from build123d import *

# Parameters (mm, degrees)
SKETCH1_R               = 32.5
BOSS_EXTRUDE1_DEPTH     = 3
CUT_EXTRUDE1_DEPTH      = 10
CUT_EXTRUDE1_DEPTH_BACK = 47.059743812
SKETCH2_W               = 5
SKETCH2_H               = 5


with BuildPart() as part:
    # Sketch1 → Boss-Extrude1 (new body)
    with BuildSketch(Plane(origin=(0, 0, 0), x_dir=(1, 0, 0), z_dir=(0, 1, 0))):
        with Locations(Location((0, 0, 0), (0, 0, 270))):
            Circle(SKETCH1_R)
    extrude(amount=BOSS_EXTRUDE1_DEPTH)

    # Sketch2 → Cut-Extrude1 (cut, two sides: drawn at the far end of the back side and taken through both)
    with BuildSketch(Plane(origin=(0, 0, 0), x_dir=(1, 0, 0), z_dir=(0, 1, 0)).offset(-CUT_EXTRUDE1_DEPTH_BACK)):
        with Locations((0, -27.5)):
            Rectangle(SKETCH2_W, SKETCH2_H)
        with Locations((27.5, 0)):
            Rectangle(SKETCH2_W, SKETCH2_H)
        with Locations((-27.5, 0)):
            Rectangle(SKETCH2_W, SKETCH2_H)
        with Locations((0, 27.5)):
            Rectangle(SKETCH2_W, SKETCH2_H)
    extrude(amount=CUT_EXTRUDE1_DEPTH + CUT_EXTRUDE1_DEPTH_BACK, mode=Mode.SUBTRACT)


solid = part.part
Geometry: final body of the model. Coordinates: model frame, mm. A direction names the side the tool comes from. Give positions to 0.01 mm unless a question says otherwise; leave off trailing zeros. Loops run counter-clockwise (first coordinate to the right, second up) from the corner with the lowest first, then second, coordinate; pieces in that order, holes last. Notation, with made-up numbers: M 42,13 L 88,13 A35 ccw 88,47 Z; hole C -11.5,32 d1. An arc over 180 degrees is marked long. Put each result on its own line as item: value. Start each with the question number.
1) Contact query for flat-ended pins moving along their axis: pin 1 (1.5 mm diameter, centred on x = -0.5, y = 1.5, fed in from +Z); pin 2 (1.5 mm diameter, centred on y = 1, z = 27.5, fed in from +X); pin 3 (1.5 mm diameter, centred on y = 1.5, z = 1, fed in from -X); pin 4 (1.5 mm diameter, centred on y = 1, z = -17, fed in from -X). Output: stop coordinate, or through.
2) Ray query, line 1 along X through (y, z) = (2.25, 0.5); line 2 along Z through (x, y) = (-25.5, 1.95); line 3 along X through (y, z) = (2.5, 26.5). Return the intervals inside material, ascending.
3) Cut plane B-B (z = 0). Output: boundary loops of the cut face in (x, y), then the cut area to 3 significant figures.
4) Cut plane D-D (z = 20.5). Output: boundary loops of the cut face in (x, y), then the cut area to 3 significant figures.
5) Cut plane A-A (x = 0). Output: boundary loops of the cut face in (y, z).
6) Pull-direction query (Z, two-part tool) for faces 1 (the flat face through (-30, 1, 0)), 2 (the cylindrical face through (9.76, 1.48, 31)), 3 (the flat face through (0, 0, 0)); classes: pulls with the +Z half, pulls with the -Z half, needs draft (parallel to the pull), parting line crosses it, or undercut.
7) Cut plane C-C (y = 1.2). Output: boundary loops of the cut face in (x, z), then the cut area to 3 significant figures.
8) Access query for faces 4 (the flat face through (2.5, 1, 28)), 5 (the flat face through (0, 3, 0)). Directions: +Z, -Z, +X, -X, +Y, -Y. A direction counts if a zero-diameter tool reaches every point of the face in a straight line with its end or side. Return the directions, or none.
Verdict:
1. pin 1: z = 32.5
1. pin 2: x = 18.46
1. pin 3: x = -32.5
1. pin 4: x = -28.15
2. line 1: -32.5 to -30, -25 to 25, 30 to 32.5
2. line 2: -20.15 to -2.5, 2.5 to 20.15
2. line 3: -18.81 to -2.5, 2.5 to 18.81
3. outline: M -32.5,0 L -30,0 L -30,3 L -32.5,3 Z; M -25,0 L 25,0 L 25,3 L -25,3 Z; M 30,0 L 32.5,0 L 32.5,3 L 30,3 Z
3. area: 165 mm2
4. outline: M -25.22,0 L 25.22,0 L 25.22,3 L -25.22,3 Z
4. area: 151 mm2
5. outline: M 0,-32.5 L 3,-32.5 L 3,-30 L 0,-30 Z; M 0,-25 L 3,-25 L 3,25 L 0,25 Z; M 0,30 L 3,30 L 3,32.5 L 0,32.5 Z
6. face 1: undercut
6. face 2: parting line crosses it
6. face 3: needs draft
7. outline: C 0,0 d65; hole M -30,-2.5 L -25,-2.5 L -25,2.5 L -30,2.5 Z; hole M -2.5,-30 L 2.5,-30 L 2.5,-25 L -2.5,-25 Z; hole M -2.5,25 L 2.5,25 L 2.5,30 L -2.5,30 Z; hole M 25,-2.5 L 30,-2.5 L 30,2.5 L 25,2.5 Z
7. area: 3,220 mm2
8. face 4: +Y, -Y
8. face 5: +Z, -Z, +X, -X, +Y
